Autodesk Inventor part; units mm, degrees
ref_plane "YZ Plane" through (0, 0, 0) normal (1, 0, 0) x (0, 1, 0)
ref_plane "XZ Plane" through (0, 0, 0) normal (0, 1, 0) x (-1, 0, 0)
ref_plane "XY Plane" through (0, 0, 0) normal (0, 0, 1) x (1, 0, 0)
sketch "スケッチ1" plane through (0, 0, 0) normal (0, 0, 1) x (1, 0, 0)
  line L0 (-50, 12) -> (50, 12)
  line L1 (50, 12) -> (50, -12)
  line L2 (50, -12) -> (-50, -12)
  line L3 (-50, -12) -> (-50, 12)
  point P0 (0, 0)
  dimension "d0" = 100
  dimension "d1" = 24
  dimension "d2" = 12
  dimension "d3" = 50
extrude "押し出し1" add sketch "スケッチ1" along normal blind 5
sketch "スケッチ2" plane through (0, 0, 5) normal (0, 0, 1) x (1, 0, 0)
  line L0 (9.2, 9.8) -> (45, 9.8)
  line L1 (45, 9.8) -> (45, -9.8)
  line L2 (45, -9.8) -> (9.2, -9.8)
  line L3 (9.2, -9.8) -> (9.2, 9.8)
  line L4 (45, 9.8) -> (40.75, 9.8)
  line L5 (40.75, 9.8) -> (40.75, -9.8)
  line L6 (40.75, -9.8) -> (45, -9.8)
  line L7 (45, -9.8) -> (45, 9.8)
  line L8 (40.75, -9.8) -> (24.75, -9.8)
  line L9 (24.75, -9.8) -> (24.75, 9.8)
  line L10 (24.75, 9.8) -> (40.75, 9.8)
  line L11 (40.75, 9.8) -> (40.75, -9.8)
  circle A0 centre (18, 0) radius 5
  line L12 (45, 0) -> (9.2, 0)
  circle A1 centre (11.8, 7.2) radius 1.25
  circle A2 centre (42.9, 7.7) radius 1.25
  circle A3 centre (11.8, -7.2) radius 1.25
  circle A4 centre (42.9, -7.7) radius 1.25
  line L13 (50, 12) -> (50, -12)
  point P0 (0, 0)
  dimension "d6" = 35.8
  dimension "d7" = 19.6
  dimension "d8" = 9.8
  dimension "d10" = 4.25
  dimension "d11" = 16
  dimension "d12" = 10
  dimension "d13" = 27
  dimension "d14" = 14.4
  dimension "d15" = 15.4
  dimension "d16" = 31.1
  dimension "d17" = 2.1
  dimension "d18" = 2.5
  dimension "d19" = 2.5
  dimension "d47" = 5
extrude "押し出し2" cut sketch "スケッチ2" against normal through all contours L0 L5 L12 L9 | L12 L5 L2 L9 | L12 A0 | A0 L12 | A1 | A2 | A3 | A4
fillet "フィレット1" radius 5 2 edges at (24.75, 9.8, 2.5) (24.75, -9.8, 2.5)
fillet "フィレット2" radius 1 2 edges at (40.75, 9.8, 2.5) (40.75, -9.8, 2.5)
sketch "スケッチ5" plane through (0, 0, 5) normal (0, 0, 1) x (1, 0, 0)
  line L0 (50, 12) -> (50, -12)
  line L1 (39.75, -9.8) -> (29.75, -9.8)
  arc A0 (24.75, -4.8) -> (29.75, -9.8) centre (29.75, -4.8) ccw
  line L2 (24.75, -4.8) -> (24.75, 4.8)
  arc A1 (29.75, 9.8) -> (24.75, 4.8) centre (29.75, 4.8) ccw
  line L3 (29.75, 9.8) -> (39.75, 9.8)
  arc A2 (40.75, 8.8) -> (39.75, 9.8) centre (39.75, 8.8) ccw
  line L4 (40.75, 8.8) -> (40.75, -8.8)
  arc A3 (39.75, -9.8) -> (40.75, -8.8) centre (39.75, -8.8) ccw
  circle A4 centre (42.9, -7.7) radius 1.25
  circle A5 centre (11.8, -7.2) radius 1.25
  circle A6 centre (42.9, 7.7) radius 1.25
  circle A7 centre (11.8, 7.2) radius 1.25
  circle A8 centre (18, 0) radius 5
  line L5 (50, 10) -> (-50, 10)
  line L6 (-50, 10) -> (-50, -10)
  line L7 (-50, -10) -> (50, -10)
  line L8 (50, -10) -> (50, 10)
  point P0 (-32.5, 14.4762)
  point P1 (-32.5, -14.4762)
  point P2 (0, 0)
  dimension "d41" = 20
  dimension "d42" = 10
  dimension "d49" = 61.8
extrude "押し出し4" cut sketch "スケッチ5" against normal blind 3
fillet "フィレット3" radius 12 4 edges at (50, -12, 2.5) (50, 12, 2.5) (-50, -12, 2.5) (-50, 12, 2.5)
fillet "フィレット4" radius 0.5 4 edges at (-44.6333, -10, 3.5) (-44.6333, 10, 3.5) (44.6333, 10, 3.5) (44.6333, -10, 3.5)
sketch "スケッチ6" plane through (0, 0, 2) normal (0, 0, 1) x (1, 0, 0)
  circle A0 centre (42.9, -7.7) radius 1.25
  circle A1 centre (36.72, 0) radius 6.5
  point P0 (0, 0)
  dimension "d52" = 13
  dimension "d53" = 6.18
extrude "押し出し5" cut sketch "スケッチ6" against normal through all contours A1
sketch "スケッチ7" plane through (0, 0, 2) normal (0, 0, 1) x (1, 0, 0)
  circle A0 centre (11.8, -7.2) radius 1.25
  circle A1 centre (11.8, 7.2) radius 1.25
  point P0 (0, 0)
  point P1 (-16.2, 7.2)
  point P2 (-16.2, -7.2)
  point P3 (-31.2, -7.2)
  point P4 (-31.2, 7.2)
  point P5 (-16.2, 7.2)
  point P6 (-31.2, 7.2)
  dimension "d56" = 15
  dimension "d57" = 15
  dimension "d58" = 28
  dimension "d59" = 28
  dimension "d60" = 7.2
  dimension "d61" = 7.2
  dimension "d62" = 7.2
  dimension "d63" = 7.2
hole "Hole2" at (-16.2, 7.2, 2) at (-16.2, -7.2, 2) at (-31.2, -7.2, 2) at (-31.2, 7.2, 2) direction (0, 0, -1) diameter 2.5 end through all
properties part number "JointC2_"
The model under review builds one solid part; all positions refer to its coordinate system, in mm. A direction names the side the tool comes from. Give positions to 0.01 mm unless a question says otherwise; leave off trailing zeros. Loops run counter-clockwise (first coordinate to the right, second up) from the corner with the lowest first, then second, coordinate; pieces in that order, holes last. Notation, with made-up numbers: (-13.75, 21) - (11.25, 21) arc R30 cw to (11.25, 48) - close; hole circle Ø1 at (55.25, 62.5). An arc over 180 degrees is marked (long way). Answer as a JSON object with one key per item and string values.
Q1. Add section B-B on z = 4.05. State the section outline as (x, y) points, plus the area to 3 significant figures.
Worked out:
{"outline": "(-42.89, -10.96) arc R12 ccw to (-38, -12) - (38, -12) arc R12 ccw to (42.89, -10.96) arc R0.5 ccw to (42.69, -10) - (-42.69, -10) arc R0.5 ccw to start; (-42.89, 10.96) arc R0.5 ccw to (-42.69, 10) - (42.69, 10) arc R0.5 ccw to (42.89, 10.96) arc R12 ccw to (38, 12) - (-38, 12) arc R12 ccw to start", "area": "337 mm^2"}
Q2. To check wall thickness, follow line 1 along Y through (x, z) = (-31.2, 0.95); line 2 along Y through (x, z) = (18, 0.4); line 3 along Y through (x, z) = (7, 3.15). State the ranges of each line that lie inside material, in increasing order.
Worked out:
{"line 1": "y = -12 to -8.45, -5.95 to 5.95, 8.45 to 12", "line 2": "y = -12 to -5, 5 to 12", "line 3": "y = -12 to -10, 10 to 12"}
Q3. Add section D-D on x = 7.5. State the section outline as (y, z) points.
Worked out:
{"outline": "(-12, 0) - (12, 0) - (12, 5) - (10, 5) - (10, 2) - (-10, 2) - (-10, 5) - (-12, 5) - close"}
Q4. For faces 1 (the flat face through (-1, -11, 5)), 2 (the flat face through (-1, -10, 4)), 3 (the cylindrical face through (43.22, -0.08, 1.01)), list the 3-axis set-ups (+Z, -Z, +X, -X, +Y, -Y) from which the entire face can be reached by the end or side of a thin tool; tool diameter is ignored.
Worked out:
{"face 1": "+Z, +X, -X, +Y, -Y", "face 2": "+Z, +X, -X", "face 3": "+Z, -Z"}
Q5. Add section C-C on y = -1.75. State the section outline as (x, z) points, plus the area to 3 significant figures.
Worked out:
{"outline": "(-49.87, 0) - (13.32, 0) - (13.32, 2) - (-49.87, 2) - close; (22.68, 0) - (24.75, 0) - (24.75, 2) - (22.68, 2) - close; (42.98, 0) - (49.87, 0) - (49.87, 2) - (42.98, 2) - close", "area": "144 mm^2"}
Q6. Insertion check: pin 1 (0.6 mm diameter, centred on y = 6.5, z = 0.5, fed in from -X); pin 2 (2 mm diameter, centred on x = 11.8, y = 7.2, fed in from +Z); pin 3 (1.6 mm diameter, centred on y = 1, z = 1, fed in from +X); pin 4 (4 mm diameter, centred on x = -31.2, y = 7.2, fed in from +Z). Each pin has a flat end and moves straight along its axis. Give the tip position at first contact, or say it passes through.
Worked out:
{"pin 1": "stops at x = -48.27", "pin 2": "passes through", "pin 3": "stops at x = 50", "pin 4": "stops at z = 2"}
Q7. Mouldability with a two-part tool opening along X and no side actions: class faces 4 (the flat face through (-1, 12, 2)), 5 (the cylindrical face through (10.81, 6.44, 1.01)), 6 (the cylindrical face through (-44.991, -9.754, 1.424)), 7 (the cylindrical face through (44.991, 9.754, 1.424)) as +X half, -X half, draft (parallel to the pull), parting line (faces both ways), or undercut.
Worked out:
{"face 4": "draft", "face 5": "undercut", "face 6": "-X half", "face 7": "+X half"}
Q8. Add section A-A on x = 18. State the section outline as (y, z) points.
Worked out:
{"outline": "(-12, 0) - (-5, 0) - (-5, 2) - (-10, 2) - (-10, 5) - (-12, 5) - close; (5, 0) - (12, 0) - (12, 5) - (10, 5) - (10, 2) - (5, 2) - close"}
